Autodesk Inventor part; units mm, degrees
ref_plane "YZ Plane" through (0, 0, 0) normal (1, 0, 0) x (0, 1, 0)
ref_plane "XZ Plane" through (0, 0, 0) normal (0, 1, 0) x (-1, 0, 0)
ref_plane "XY Plane" through (0, 0, 0) normal (0, 0, 1) x (1, 0, 0)
sketch "Sketch1" plane through (0, 0, 0) normal (0, 1, 0) x (-1, 0, 0)
  line L0 (63.4999, 10.16) -> (-63.4999, 10.16)
  line L1 (-63.5, -10.16) -> (63.5, -10.16)
  line L2 (63.4999, 10.16) -> (-63.5, -10.16) construction
  line L3 (-63.4999, 10.16) -> (63.5, -10.16) construction
  line L4 (-63.5, -7.62) -> (-50.8, -7.62)
  line L5 (-50.8, -7.62) -> (-50.8, 0)
  line L6 (0, 0) -> (-63.5, 0.0004) construction
  line L7 (0, 0) -> (0, -10.16) construction
  line L8 (-63.4999, 7.6208) -> (-50.7999, 7.6206)
  line L9 (-50.7999, 7.6206) -> (-50.8, 0)
  line L10 (63.5, -7.62) -> (50.8, -7.62)
  line L11 (50.8, -7.62) -> (50.8, 0)
  line L12 (63.4999, 7.6208) -> (50.7999, 7.6206)
  line L13 (50.7999, 7.6206) -> (50.8, 0)
  line L14 (63.5, -10.16) -> (63.5, -7.62)
  line L15 (63.4999, 7.6208) -> (63.4999, 10.16)
  line L16 (-63.4999, 10.16) -> (-63.4999, 7.6208)
  line L17 (-63.5, -7.62) -> (-63.5, -10.16)
  dimension "length" = 127
  dimension "oneHalfCutoffWidth" = 7.62
  dimension "cutoutWidth" = 12.7
  dimension "width" = 20.32
extrude "Extrusion1" add sketch "Sketch1" along normal mid plane 6.35
sketch "Sketch2" plane through (-63.4999, 3.175, 10.16) normal (0, 0, 1) x (1, 0, 0)
  line L0 (63.4999, -3.175) -> (63.4999, 0) construction
  line L1 (0, 0) -> (126.9998, 0) construction
  point P0 (122.8089, -3.175)
  point P1 (4.1909, -3.175)
  dimension "d8" = 59.309
hole "Hole1" at (59.309, 0, 10.16) at (-59.309, 0, 10.16) direction (0, 0, -1) diameter 3.2766 end through all
fillet "Fillet2" radius 3.175 8 edges at (63.5, 3.175, -8.89) (63.5, -3.175, -8.89) (63.4999, 3.175, 8.8904) (63.4999, -3.175, 8.8904) (-63.4999, 3.175, 8.8904) (-63.4999, -3.175, 8.8904) (-63.5, 3.175, -8.89) (-63.5, -3.175, -8.89)
sketch "Sketch5" plane through (0, 3.175, 0) normal (0, 1, 0) x (1, 0, 0)
  line L0 (-50.8, 0) -> (50.8, 0) construction
  line L1 (-34.4338, 6.35) -> (-30.7677, 0)
  line L2 (-30.7677, 0) -> (-34.4338, -6.35)
  line L3 (-34.4338, -6.35) -> (-41.7662, -6.35)
  line L4 (-41.7662, -6.35) -> (-45.4323, 0)
  line L5 (-45.4323, 0) -> (-41.7662, 6.35)
  line L6 (-41.7662, 6.35) -> (-34.4338, 6.35)
  line L7 (-50.8, 0) -> (-50.7999, -7.6206)
  line L8 (-16.3662, 6.35) -> (-9.0338, 6.35)
  line L9 (-9.0338, 6.35) -> (-5.3677, 0)
  line L10 (-5.3677, 0) -> (-9.0338, -6.35)
  line L11 (-9.0338, -6.35) -> (-16.3662, -6.35)
  line L12 (-16.3662, -6.35) -> (-20.0323, 0)
  line L13 (-20.0323, 0) -> (-16.3662, 6.35)
  line L14 (9.0338, 6.35) -> (16.3662, 6.35)
  line L15 (16.3662, 6.35) -> (20.0323, 0)
  line L16 (20.0323, 0) -> (16.3662, -6.35)
  line L17 (16.3662, -6.35) -> (9.0338, -6.35)
  line L18 (9.0338, -6.35) -> (5.3677, 0)
  line L19 (5.3677, 0) -> (9.0338, 6.35)
  line L20 (34.4338, 6.35) -> (41.7662, 6.35)
  line L21 (41.7662, 6.35) -> (45.4323, 0)
  line L22 (45.4323, 0) -> (41.7662, -6.35)
  line L23 (41.7662, -6.35) -> (34.4338, -6.35)
  line L24 (34.4338, -6.35) -> (30.7677, 0)
  line L25 (30.7677, 0) -> (34.4338, 6.35)
  point P0 (0, 0)
  point P1 (-38.1, 0)
  dimension "d18" = 12.7
  dimension "d19" = 12.7
  dimension "d22" = 25.4
extrude "Extrusion2" cut sketch "Sketch5" against normal through all
equation "\"endFilet\" = 0.5 * depth"
properties part number "supportPiece"
Geometry: final body of the model. Coordinates: model frame, mm. A direction names the side the tool comes from. Give positions to 0.01 mm unless a question says otherwise; leave off trailing zeros. Loops run counter-clockwise (first coordinate to the right, second up) from the corner with the lowest first, then second, coordinate; pieces in that order, holes last. Notation, with made-up numbers: (52, 14.25) -> (93, 14.25) arc R5 cw to (93, 23.25) -> close; hole circle Ø3 at (80, -19.75). An arc over 180 degrees is marked (long way). Return JSON: item names as keys, results as strings.
Item 1: Mould query, pull axis X, two halves, no side actions, for faces 3 (the flat face through (43.625, 0.044, 3.131)), 4 (the cylindrical face through (-62.545, 2.27, 8.908)), 5 (the flat face through (57, 0, -7.62)), 6 (the cylindrical face through (62.595, -2.22, 8.873)). Classes: released by +X, released by -X, zero draft, split by the parting line, or undercut.
Filled in:
{"face 3": "undercut", "face 4": "released by -X", "face 5": "zero draft", "face 6": "released by +X"}
Item 2: Pin query (flat end, axial travel): P1, Ø1.5, axis at y = -0.5, z = -4, coming from the +X side; P2, Ø2, axis at y = -2.5, z = -4, coming from the -X side. Return the tip coordinate at first contact, or that it passes through.
Filled in:
{"P1": "x = 50.8", "P2": "x = -50.8"}
Item 3: Line query: line 1 (X direction, y = 0, z = -9.3); line 2 (X direction, y = -1.5, z = -5); line 3 (X direction, y = -2.5, z = -4.75). Output: solid intervals per line, ascending.
Filled in:
{"line 1": "-63.5 to -60.95, -57.67 to 57.67, 60.95 to 63.5", "line 2": "-50.8 to -42.55, -33.65 to -17.15, -8.25 to 8.25, 17.15 to 33.65, 42.55 to 50.8", "line 3": "-50.8 to -42.69, -33.51 to -17.29, -8.11 to 8.11, 17.29 to 33.51, 42.69 to 50.8"}
Item 4: Section B-B, the plane x = 33. Output: boundary loops of the cut face in (y, z) (3 decimals), plus the area to 3 significant figures.
Filled in:
{"outline": "(-3.175, -10.16) -> (3.175, -10.16) -> (3.175, -3.867) -> (-3.175, -3.867) -> close; (-3.175, 3.867) -> (3.175, 3.867) -> (3.175, 10.16) -> (-3.175, 10.16) -> close", "area": "79.9 mm^2"}
Item 5: Access query for faces 1 (the cylindrical face through (62.545, 2.27, -8.908)), 2 (the flat face through (-38, 0, -6.35)). Directions: +Z, -Z, +X, -X, +Y, -Y. A direction counts if a zero-diameter tool reaches every point of the face in a straight line with its end or side. Return the directions, or none.
Filled in:
{"face 1": "+Z, -Z, +X, +Y", "face 2": "+Y, -Y"}
Item 6: Section A-A, the plane x = -35.5. Output: boundary loops of the cut face in (y, z) (3 decimals), plus the area to 3 significant figures.
Filled in:
{"outline": "(-3.175, -10.16) -> (3.175, -10.16) -> (3.175, -6.35) -> (-3.175, -6.35) -> close; (-3.175, 6.35) -> (3.175, 6.35) -> (3.175, 10.16) -> (-3.175, 10.16) -> close", "area": "48.4 mm^2"}
